Source: CAD feature listing. Evaluate the final solid. Frame: model axes, mm. A direction names the side the tool comes from. Give positions to 0.01 mm unless a question says otherwise; leave off trailing zeros. Order: outer loops, then holes, each group sorted by start corner. A loop starts at its lowest first (then second) coordinate and runs counter-clockwise, first axis right, second up. Notation, with made-up numbers: M 23,56 L 41,56 A13 ccw 41,76 Z; hole C 56.25,10.5 d1. An arc over 180 degrees is marked long. Answer in a Markdown table with one row per item. Add a question column.
(1) Material intervals for line 1 along Y through (x, z) = (-10.25, 7.5) (3 decimals); line 2 along X through (y, z) = (6, 2.5); line 3 along Y through (x, z) = (-12.25, 14), sorted ascending.
(2) Pin query (flat end, axial travel): P1, Ø4, axis at y = 21.5, z = 8, coming from the -X side; P2, Ø11, axis at x = -10.74, y = -26.57, coming from the +Z side; P3, Ø0.9, axis at y = 28, z = 6, coming from the +X side; P4, Ø0.5, axis at y = 27.5, z = 8.5, coming from the -X side. Return the tip coordinate at first contact, or that it passes through.
(3) Section query D-D, the plane x = 0.75. Return loops of the section in (y, z), plus the area to 3 significant figures.
(4) Section query A-A, the plane x = -7. Return loops of the section in (y, z), plus the area to 3 significant figures.
(5) Mould query, pull axis X, two halves, no side actions, for faces 1 (the face through (-9.55, -26.49, 19.622)), 2 (the face through (-3.166, 16.3, 3.1)), 3 (the face through (-7.22, 7.66, 2.35)). Classes: pulls with the +X half, pulls with the -X half, needs draft (parallel to the pull), parting line crosses it, or undercut.
(6) Section query C-C, the plane z = 18.25. Return loops of the section in (x, y) (3 decimals), plus the area to 3 significant figures.
(7) Section query B-B, the plane y = -2. Return loops of the section in (x, z).
(8) Set-up query: faces 4 (the face through (-2.806, 12, 2)), 5 (the face through (-10.7, 30.4, 12.7)), 6 (the face through (-9.727, -27, 12)). Return all of +Z, -Z, +X, -X, +Y, -Y with unobstructed straight access to the full face (end or side cutting, diameter ignored); none if empty.
from build123d import *

# Parameters (mm, degrees)
SKETCH1_R           = 7.880311683
SKETCH1_R_2         = 1.7907
SKETCH1_R_3         = 4.746605842
BOSS_EXTRUDE1_DEPTH = 12.7
SKETCH5_W           = 7.9375
SKETCH5_H           = 27.701129001
SKETCH5_H_2         = 7.880311683
CUT_EXTRUDE1_DEPTH  = 43.908371508
SKETCH6_R           = 5.715
BOSS_EXTRUDE2_DEPTH = 14.859


with BuildPart() as part:
    # Sketch1 → Boss-Extrude1 (new body)
    # profile 1 of 4: a face of its own
    with BuildSketch(Plane.XY):
        with Locations((-10.68587239, -26.593250225)):
            Circle(SKETCH1_R)
    # profile 2 of 4: a face of its own
    with BuildSketch(Plane.XY):
        with BuildLine():
            Line((3.60162761, 11.531317118), (-2.805560707, 11.531317118))
            Line((-2.805560707, 11.531317118), (-18.566184073, 11.531317118))
            Line((-18.566184073, 11.531317118), (-18.566184073, -26.593250225))
            ThreePointArc((-18.566184073, -26.593250225), (-10.68587239, -18.712938542), (-2.805560707, -26.593250225))
            Line((-2.805560707, -26.593250225), (-2.805560707, 1.359449775))
            Line((-2.805560707, 1.359449775), (3.60162761, 1.359449775))
            Line((3.60162761, 1.359449775), (3.60162761, 11.531317118))
        make_face()
        with Locations((-10.628684073, -13.868682882)):
            Circle(SKETCH1_R_2, mode=Mode.SUBTRACT)
        with Locations((-5.89797239, 6.451317118)):
            Circle(SKETCH1_R_2, mode=Mode.SUBTRACT)
        with Locations((-0.151184073, 6.451317118)):
            Circle(SKETCH1_R_2, mode=Mode.SUBTRACT)
    # profile 3 of 4: a face of its own
    with BuildSketch(Plane.XY):
        with BuildLine():
            Line((-5.89797239, 27.24757345), (-5.89797239, 28.334249775))
            ThreePointArc((-5.89797239, 28.334249775), (-10.644578231, 23.587643933), (-15.391184073, 28.334249775))
            Line((-15.391184073, 28.334249775), (-15.391184073, 27.2867057))
            ThreePointArc((-15.391184073, 27.2867057), (-15.767187067, 23.64949685), (-16.879292984, 20.16612393))
            Line((-16.879292984, 20.16612393), (-17.078075162, 19.711310306))
            ThreePointArc((-17.078075162, 19.711310306), (-18.190181079, 16.227937386), (-18.566184073, 12.590728536))
            Line((-18.566184073, 12.590728536), (-18.566184073, 11.531317118))
            Line((-18.566184073, 11.531317118), (-2.805560707, 11.531317118))
            Line((-2.805560707, 11.531317118), (-2.805560707, 12.738028185))
            ThreePointArc((-2.805560707, 12.738028185), (-3.176236758, 16.349653807), (-4.272809259, 19.810689652))
            Line((-4.272809259, 19.810689652), (-4.430723837, 20.174911983))
            ThreePointArc((-4.430723837, 20.174911983), (-5.527296339, 23.635947828), (-5.89797239, 27.24757345))
        make_face()
    # profile 4 of 4: a face of its own
    with BuildSketch(Plane.XY):
        with Locations((-10.644578231, 28.334249775)):
            Circle(SKETCH1_R_3)
        with Locations((-10.644578231, 28.334249775)):
            Circle(SKETCH1_R_2, mode=Mode.SUBTRACT)
    extrude(amount=BOSS_EXTRUDE1_DEPTH)

    # Sketch5 → Cut-Extrude1 (cut, through all)
    with BuildSketch(Plane.ZY.offset(18.566184073)):
        Polygon((4.7625, 11.267878776), (4.7625, 1.107878776), (12.7, 1.107878776), (12.7, 12.590728536), (4.7625, 12.590728536), align=None)
        with BuildLine():
            Line((4.7625, 12.590728536), (12.7, 12.590728536))
            Line((12.7, 12.590728536), (12.7, 27.644937325))
            ThreePointArc((12.7, 27.644937325), (11.790590228, 23.757613113), (9.251115022, 20.677129167))
            Line((9.251115022, 20.677129167), (8.211384978, 19.88416172))
            ThreePointArc((8.211384978, 19.88416172), (5.671909772, 16.803677773), (4.7625, 12.916353561))
            Line((4.7625, 12.916353561), (4.7625, 12.590728536))
        make_face()
        with Locations((8.73125, -12.742685725)):
            Rectangle(SKETCH5_W, SKETCH5_H)
        with Locations((8.73125, -30.533406066)):
            Rectangle(SKETCH5_W, SKETCH5_H_2)
    extrude(amount=-CUT_EXTRUDE1_DEPTH, mode=Mode.SUBTRACT)

    # Sketch6 → Boss-Extrude2 (add)
    with BuildSketch(Plane.XY.offset(4.7625)):
        with Locations((-10.743060707, -26.568682882)):
            Circle(SKETCH6_R)
        with BuildLine():
            Line((-9.727060707, -23.293658454), (-9.727060707, -29.843707309))
            ThreePointArc((-9.727060707, -29.843707309), (-14.172060707, -26.568682882), (-9.727060707, -23.293658454))
        make_face(mode=Mode.SUBTRACT)
    extrude(amount=BOSS_EXTRUDE2_DEPTH)


solid = part.part
Values follow:
| question | item | result |
|---|---|---|
| 1 | line 1 | y = -32.262 to -29.962, -23.175 to -20.875, 19.279 to 26.588, 30.081 to 33.064 |
| 1 | line 2 | x = -18.57 to -7.63, -4.17 to -1.88, 1.58 to 3.6 |
| 1 | line 3 | y = -32.08 to -29.65, -23.49 to -21.06 |
| 2 | P1 | stops at x = -17.16 |
| 2 | P2 | stops at z = 19.62 |
| 2 | P3 | stops at x = -5.9 |
| 2 | P4 | stops at x = -15.39 |
| 3 | outline | M 1.36,0 L 4.9,0 L 4.9,4.76 L 1.36,4.76 Z; M 8,0 L 11.53,0 L 11.53,4.76 L 8,4.76 Z |
| 3 | area | 33.7 mm² |
| 4 | outline | M -33.56,0 L 5.04,0 L 5.04,4.76 L -22.25,4.76 L -22.25,19.62 L -30.89,19.62 L -30.89,4.76 L -33.56,4.76 Z; M 7.86,0 L 31.38,0 L 31.38,12.7 L 27.64,12.7 A8.76 ccw 20.68,9.25 L 19.88,8.21 A8.76 cw 12.92,4.76 L 7.86,4.76 Z |
| 4 | area | 512 mm² |
| 5 | face 1 | needs draft |
| 5 | face 2 | pulls with the +X half |
| 5 | face 3 | undercut |
| 6 | outline | C -10.743,-26.569 d11.43; hole M -9.727,-29.844 L -9.727,-23.294 A3.429 ccw long Z |
| 6 | area | 77.3 mm² |
| 7 | outline | M -18.57,0 L -2.81,0 L -2.81,4.76 L -18.57,4.76 Z |
| 8 | face 4 | +Z, -Z, +X, +Y |
| 8 | face 5 | +Z, +X, -X, +Y |
| 8 | face 6 | +Z |
